Source: CAD feature listing. Evaluate the final solid. Frame: model axes, mm. Face numbers are marked on the shaded views. A direction names the side the tool comes from. Round coordinates to 2 decimals unless told otherwise and drop trailing zeros. Order: outer loops, then holes, each group sorted by start corner. A loop starts at its lowest first (then second) coordinate and runs counter-clockwise, first axis right, second up. Notation, with made-up numbers: M -11,31 L 6,31 A28 cw 6,66 Z; hole C -25,25 d11. An arc over 180 degrees is marked long. Answer as CSV lines item,"result". Start each with the question number.
Item 1: Pull-direction query (X, two-part tool) for the marked faces 1, 2 and 3; classes: +X half, -X half, draft (parallel to the pull), parting line (faces both ways), or undercut.
Item 2: Line query: line 1 (Y direction, x = -6, z = 13); line 2 (Z direction, x = 61, y = -23.5); line 3 (Z direction, x = 37, y = -52) (3 decimals). Output: solid intervals per line, ascending. Write a range as [from, to].
Item 3: Set-up query: the marked faces 4, 5 and 6. Return all of +Z, -Z, +X, -X, +Y, -Y with unobstructed straight access to the full face (end or side cutting, diameter ignored); none if empty.
Item 4: Section query A-A on x = 81.5. Return the cut outline in (y, z) (3 decimals).
Item 5: Section query B-B on y = -17. Return the cut outline in (x, z) (3 decimals).
Item 6: Section query C-C on y = -40. Return the cut outline in (x, z) (3 decimals), plus the area to 3 significant figures.
Item 7: First-contact query: P1, Ø1.5, axis at y = -13, z = 28.5, coming from the -X side; P2, Ø1, axis at x = 13.5, y = 48.5, coming from the +Z side (3 decimals); P3, Ø1.5, axis at y = -16, z = 41.5, coming from the -X side. Flat tips, straight axial feed; report the tip coordinate or a pass-through.
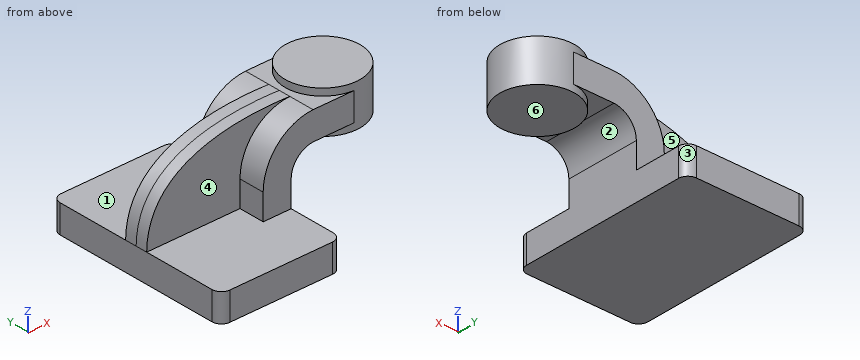
from build123d import *

# Parameters (mm, degrees)
F1_DEPTH = 63.5
F2_DEPTH = 25.4
F3_DEPTH = 7.9375
F0_W     = 25.3550079346
F0_H     = 19.05
F5_DEPTH = 25.4
F6_R     = 6.35


with BuildPart() as f1:
    # F0 (on Front) → F1 (new body, symmetric)
    with BuildSketch(Plane.XZ):
        Polygon((-41.275, -9.525), (41.275, -9.525), (41.275, 9.525), (22.225, 9.525), (-41.275, 9.525), align=None)
    extrude(amount=F1_DEPTH, both=True)

    # F0 (on Front) → F2 (join, symmetric)
    with BuildSketch(Plane.XZ):
        with BuildLine():
            Line((22.225, 9.525), (41.275, 9.525))
            Line((41.275, 9.525), (41.275, 27.0139750475))
            ThreePointArc((41.275, 27.0139750475), (45.6932996526, 38.0030442596), (56.4888131842, 42.8752))
            Line((56.4888131842, 42.8752), (60.325, 42.8752))
            Line((60.325, 42.8752), (60.325, 61.9252))
            Line((60.325, 61.9252), (56.1691853824, 61.9252))
            ThreePointArc((56.1691853824, 61.9252), (32.1099263627, 51.3604396212), (22.225, 27.0139750475))
            Line((22.225, 27.0139750475), (22.225, 9.525))
        make_face()
    extrude(amount=F2_DEPTH, both=True)

    # F0 (on Front) → F3 (join, symmetric)
    with BuildSketch(Plane.XZ):
        with BuildLine():
            add(Edge.make_bspline(
                [(-41.275, 9.525), (-40.7000668347, 58.4918707609), (18.3322690427, 63.7783482671), (56.1691853824, 61.9252)],
                knots=[0, 0, 0, 0, 110.6397316739, 110.6397316739, 110.6397316739, 110.6397316739], degree=3))
            Line((-41.275, 9.525), (22.225, 9.525))
            Line((22.225, 9.525), (22.225, 27.0139750475))
            ThreePointArc((22.225, 27.0139750475), (32.1099263627, 51.3604396212), (56.1691853824, 61.9252))
        make_face()
    extrude(amount=F3_DEPTH, both=True)

    # F0 (on Front) → F4 (revolve)
    with BuildSketch(Plane.XZ):
        Polygon((85.6800079346, 66.675), (85.6800079346, 61.9252), (85.7112655525, 61.9252), (85.7112655525, 42.8752), (85.6800079346, 42.8752), (85.6800079346, 38.1), (111.125, 38.1), (111.125, 66.675), align=None)
    revolve(axis=Axis((85.6800079346, 0, 52.3875), (0, 0, 1)))

    # F0 (on Front) → F5 (join, symmetric)
    with BuildSketch(Plane.XZ):
        with Locations((73.0025039673, 52.4002)):
            Rectangle(F0_W, F0_H)
    extrude(amount=F5_DEPTH, both=True)

    # F6
    f6_edges = [f1.edges().sort_by_distance(p)[0] for p in [
        (41.275, -63.5, 0),
        (-41.275, -63.5, 0),
        (41.275, 63.5, 0),
        (-41.275, 63.5, 0),
    ]]
    fillet(f6_edges, radius=F6_R)


solid = f1.part
Results:
1,face 1,"draft"
1,face 2,"undercut"
1,face 3,"+X half"
2,line 1,"[-7.94, 7.94]"
2,line 2,"[42.88, 61.93]"
2,line 3,"[-9.525, 9.525]"
3,face 4,"+Z, -X, -Y"
3,face 5,"+Z, -X, +Y"
3,face 6,"-Z, +X, +Y, -Y"
4,outline,"M -25.4,42.875 L -25.099,42.875 L -25.099,38.1 L 25.099,38.1 L 25.099,42.875 L 25.4,42.875 L 25.4,61.925 L 25.099,61.925 L 25.099,66.675 L -25.099,66.675 L -25.099,61.925 L -25.4,61.925 Z"
5,outline,"M -41.275,-9.525 L 41.275,-9.525 L 41.275,27.014 A15.875 cw 56.489,42.875 L 66.747,42.875 L 66.747,38.1 L 104.613,38.1 L 104.613,66.675 L 66.747,66.675 L 66.747,61.925 L 56.169,61.925 A34.925 ccw 22.225,27.014 L 22.225,9.525 L -41.275,9.525 Z"
6,outline,"M -41.275,-9.525 L 41.275,-9.525 L 41.275,9.525 L -41.275,9.525 Z"
6,area,"1,570 mm^2"
7,P1,"x = 22.23"
7,P2,"z = 9.525"
7,P3,"x = 25.04"
